Part model, mm, in its own coordinate system. Round coordinates to 2 decimals unless told otherwise and drop trailing zeros. Write each loop counter-clockwise with the first axis right and the second up, starting at its lowest first coordinate (ties: lowest second). Pieces come first, ordered by that corner, then holes. Notation, with made-up numbers: M -3.5,-2.75 L 15.5,-2.75 A21 cw 15.5,24.25 Z; hole C 3,-0.75 d8. An arc over 180 degrees is marked long. Use a Markdown table: item, result. Add a question column.
1) Slice it at C-C on x = 371. Write the cut outline in (y, z).
2) Wall check: probe 1 along Y at (x, z) = (249, 0.75); probe 2 along X at (y, z) = (45.5, 0.85); probe 3 along Y at (x, z) = (204.5, 0.85). Give the ranges that are in metal, low to high.
3) Slice it at B-B on y = -44. Write the cut outline in (x, z).
4) Slice it at A-A on z = 0.4. Write the cut outline in (x, y), plus the area to 3 significant figures.
```python
from build123d import *

# Parameters (mm, degrees)
LINEAR_AUSTRAGEN1_DEPTH = 1


with BuildPart() as part:
    # Skizze1 → Linear austragen1 (new body)
    with BuildSketch(Plane.XY):
        with BuildLine():
            Line((0, 50), (200, 50))
            Line((200, 50), (200, 35))
            ThreePointArc((200, 35), (202.928932188, 27.928932188), (210, 25))
            Line((210, 25), (400, 25))
            Line((400, 25), (400, -25))
            Line((400, -25), (210, -25))
            ThreePointArc((210, -25), (202.928932188, -27.928932188), (200, -35))
            Line((200, -35), (200, -50))
            Line((200, -50), (0, -50))
            Line((0, -50), (0, 50))
        make_face()
    extrude(amount=LINEAR_AUSTRAGEN1_DEPTH)


solid = part.part
```
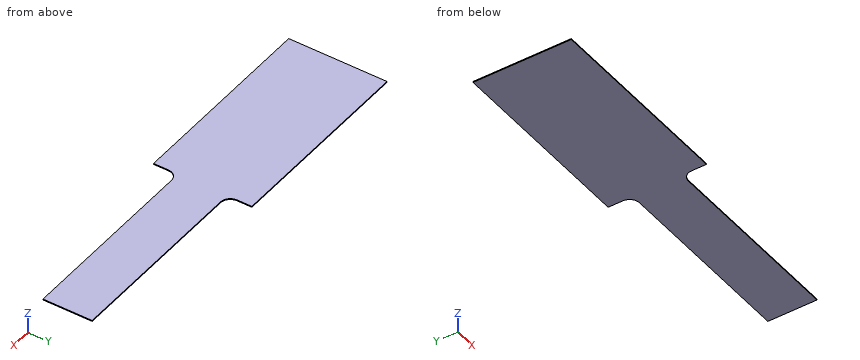
Entries:
| question | item | result |
|---|---|---|
| 1 | outline | M -25,0 L 25,0 L 25,1 L -25,1 Z |
| 2 | probe 1 | y = -25 to 25 |
| 2 | probe 2 | x = 0 to 200 |
| 2 | probe 3 | y = -26.65 to 26.65 |
| 3 | outline | M 0,0 L 200,0 L 200,1 L 0,1 Z |
| 4 | outline | M 0,-50 L 200,-50 L 200,-35 A10 cw 210,-25 L 400,-25 L 400,25 L 210,25 A10 cw 200,35 L 200,50 L 0,50 Z |
| 4 | area | 30,000 mm^2 |
